Can you work these out from the model? Positions are in its coordinate system, mm. Round coordinates to 2 decimals unless told otherwise and drop trailing zeros. Write each loop counter-clockwise with the first axis right and the second up, starting at its lowest first coordinate (ties: lowest second). Pieces come first, ordered by that corner, then holes. Notation, with made-up numbers: (72, 43) -> (102, 43) arc R24 cw to (102, 68) -> close; hole circle Ø3 at (18, 41.25). An arc over 180 degrees is marked (long way). Write item = value, one per line. Start each with the question number.
1) I'm going to push flat-ended pins straight in: pin 1 (1.5 mm diameter, centred on x = 32.91, y = 19, fed in from +Z); pin 2 (3 mm diameter, centred on x = -32.91, y = -19, fed in from +Z); pin 3 (1 mm diameter, centred on y = 21, z = 0.5, fed in from -X). Where does each tip first touch, or does it pass through?
2) Imagine slicing it at B-B, the plane x = 0. Please give me the cut outline in (y, z).
3) If I drill on line 1 (Y direction, x = 0, z = 1.25); line 2 (X direction, y = 1, z = 0.55); line 3 (Y direction, x = -18, z = 0.9), over which ranges is the centre line in solid material (lowest first)?
4) Imagine slicing it at A-A, the plane y = 0. Please give me the cut outline in (x, z).
5) Imagine slicing it at C-C, the plane x = 21. Please give me the cut outline in (y, z), then the cut area to 3 significant figures.
6) Imagine slicing it at D-D, the plane y = -19. Please give me the cut outline in (x, z), then the cut area to 3 significant figures.
7) Thinking about a two-plate mould opening in X: for faces 1 (the face through (-33.727, -25.861, 0.986)), 2 (the face through (-0.577, -36.891, 1.014)), 3 (the face through (0, 35, 0)), which applies, +X half, -X half, draft (parallel to the pull), parting line (faces both ways), or undercut?
from build123d import *

# Parameters (mm, degrees)
SKETCH_1_R                 = 42.5
SKETCH_1_R_2               = 34.5
EXTRUDE_336_DEPTH          = 2
SKETCH_3_R                 = 1.25
CUT_EXTRUDE_486_DEPTH      = 61.137342808
PATTERN_CIRCULAR_525_COUNT = 6


with BuildPart() as part:
    # Эскиз1 → Extrude 336 (new body)
    with BuildSketch(Plane.XY):
        Circle(SKETCH_1_R)
        Circle(SKETCH_1_R_2, mode=Mode.SUBTRACT)
    extrude(amount=EXTRUDE_336_DEPTH)

    # Эскиз3 → Cut-Extrude 486 (cut, through all)
    with BuildSketch(Plane.XY.offset(2)):
        with Locations((0, 38)):
            Circle(SKETCH_3_R)
    cut_extrude_486 = extrude(amount=-CUT_EXTRUDE_486_DEPTH, mode=Mode.SUBTRACT)

    # Pattern Circular 525: Cut-Extrude 486 ×6 about axis
    pattern_circular_525_axis = Axis((0, 0, 0), (0, 0, 1))
    for i in range(1, PATTERN_CIRCULAR_525_COUNT):
        add(cut_extrude_486.rotate(pattern_circular_525_axis, i * 360 / PATTERN_CIRCULAR_525_COUNT), mode=Mode.SUBTRACT)


solid = part.part
Reported:
q1.pin_1 = through
q1.pin_2 = 2
q1.pin_3 = -37.23
q2.outline = (-42.5, 0) -> (-39.25, 0) -> (-39.25, 2) -> (-42.5, 2) -> close; (-36.75, 0) -> (-34.5, 0) -> (-34.5, 2) -> (-36.75, 2) -> close; (34.5, 0) -> (36.75, 0) -> (36.75, 2) -> (34.5, 2) -> close; (39.25, 0) -> (42.5, 0) -> (42.5, 2) -> (39.25, 2) -> close
q3.line_1 = -42.5 to -39.25, -36.75 to -34.5, 34.5 to 36.75, 39.25 to 42.5
q3.line_2 = -42.49 to -34.49, 34.49 to 42.49
q3.line_3 = -38.5 to -29.43, 29.43 to 38.5
q4.outline = (-42.5, 0) -> (-34.5, 0) -> (-34.5, 2) -> (-42.5, 2) -> close; (34.5, 0) -> (42.5, 0) -> (42.5, 2) -> (34.5, 2) -> close
q5.outline = (-36.95, 0) -> (-27.37, 0) -> (-27.37, 2) -> (-36.95, 2) -> close; (27.37, 0) -> (36.95, 0) -> (36.95, 2) -> (27.37, 2) -> close
q5.area = 38.3 mm²
q6.outline = (-38.02, 0) -> (-34.16, 0) -> (-34.16, 2) -> (-38.02, 2) -> close; (-31.66, 0) -> (-28.8, 0) -> (-28.8, 2) -> (-31.66, 2) -> close; (28.8, 0) -> (31.66, 0) -> (31.66, 2) -> (28.8, 2) -> close; (34.16, 0) -> (38.02, 0) -> (38.02, 2) -> (34.16, 2) -> close
q6.area = 26.9 mm²
q7.face_1 = parting line
q7.face_2 = undercut
q7.face_3 = draft
